Geometry check sheet. Reference: the model listing, model coordinates, mm. A direction names the side the tool comes from. Coordinates: 2 decimals unless noted, no trailing zeros. Loops run counter-clockwise (first coordinate to the right, second up) from the corner with the lowest first, then second, coordinate; pieces in that order, holes last. Notation, with made-up numbers: (32.5, 87.5) -> (56.5, 87.5) arc R8 ccw to (56.5, 95.5) -> close; hole circle Ø4 at (16.25, 16.25). An arc over 180 degrees is marked (long way). Answer as a JSON object with one key per item and string values.
from build123d import *

# Parameters (mm, degrees)
F0_W     = 33.688
F0_H     = 15
F0_W_2   = 32.188
F0_H_2   = 13.5
F1_DEPTH = 3.5
F0_W_3   = 43.688
F0_H_3   = 25
F2_DEPTH = 2


with BuildPart() as f1:
    # F0 (on Front) → F1 (new body)
    with BuildSketch(Plane.XZ):
        with Locations((16.844, -7.5)):
            Rectangle(F0_W, F0_H)
        with Locations((16.844, -7.5)):
            Rectangle(F0_W_2, F0_H_2, mode=Mode.SUBTRACT)
    extrude(amount=F1_DEPTH)

    # F0 (on Front) → F2 (join)
    with BuildSketch(Plane.XZ):
        with Locations((16.844, -7.5)):
            Rectangle(F0_W_3, F0_H_3)
        with Locations((16.844, -7.5)):
            Rectangle(F0_W, F0_H, mode=Mode.SUBTRACT)
    extrude(amount=F2_DEPTH)


solid = f1.part
1. Section check A-A, the plane y = -1.15. Record the boundary of the cut face in (x, z), then the cut area to 3 significant figures.
Evaluation:
{"outline": "(-5, -20) -> (38.69, -20) -> (38.69, 5) -> (-5, 5) -> close; hole (0.75, -14.25) -> (32.94, -14.25) -> (32.94, -0.75) -> (0.75, -0.75) -> close", "area": "658 mm^2"}
2. Section check D-D, the plane z = 1.25. Record the boundary of the cut face in (x, y), then the cut area to 3 significant figures.
Evaluation:
{"outline": "(-5, -2) -> (38.69, -2) -> (38.69, 0) -> (-5, 0) -> close", "area": "87.4 mm^2"}
3. Mould release check, pull along X, two halves, no side actions. Record for faces 1 (the face through (38.688, -1, -8)), 2 (the face through (0, -3, -8)), 3 (the face through (0.75, -2, -8)), 4 (the face through (15.5, -3.5, -14.7)): released by +X, released by -X, zero draft, split by the parting line, or undercut.
Evaluation:
{"face 1": "released by +X", "face 2": "released by -X", "face 3": "undercut", "face 4": "zero draft"}
4. Depth check by flat-ended pin: P1, Ø1.2, axis at y = -3, z = -6.5, coming from the -X side. Enter the tip coordinate at first touch or a pass-through.
Evaluation:
{"P1": "stops at x = 0"}
5. Tool access check on faces 5 (the face through (33.688, -3, -8)), 6 (the face through (17, -2, -0.75)), 7 (the face through (17, -3, -15)). Record the directions out of +Z, -Z, +X, -X, +Y, -Y that give a thin tool (end or side, any length) a straight path to the whole face; none if there is none.
Evaluation:
{"face 5": "+Z, -Z, +X, -Y", "face 6": "+Y, -Y", "face 7": "-Z, +X, -X, -Y"}
6. Thickness scan on probe 1 along Z at (x, y) = (30, -0.95); probe 2 along X at (y, z) = (-2.85, -14); probe 3 along Z at (x, y) = (20.5, -2.5). Record the ranges inside material, lowest first. Write a range as from..to.
Evaluation:
{"probe 1": "z = -20..-14.25, -0.75..5", "probe 2": "x = 0..0.75, 32.94..33.69", "probe 3": "z = -15..-14.25, -0.75..0"}
7. Section check B-B, the plane z = -3. Record the boundary of the cut face in (x, y).
Evaluation:
{"outline": "(-5, -2) -> (0, -2) -> (0, -3.5) -> (0.75, -3.5) -> (0.75, 0) -> (-5, 0) -> close; (32.94, -3.5) -> (33.69, -3.5) -> (33.69, -2) -> (38.69, -2) -> (38.69, 0) -> (32.94, 0) -> close"}
8. Section check C-C, the plane x = 1.5. Record the boundary of the cut face in (y, z), then the cut area to 4 significant figures.
Evaluation:
{"outline": "(-3.5, -15) -> (-2, -15) -> (-2, -20) -> (0, -20) -> (0, -14.25) -> (-3.5, -14.25) -> close; (-3.5, -0.75) -> (0, -0.75) -> (0, 5) -> (-2, 5) -> (-2, 0) -> (-3.5, 0) -> close", "area": "25.25 mm^2"}
